Build history of the part. All positions in model axes, mm. Face numbers are marked on the shaded views. A direction names the side the tool comes from. Round coordinates to 2 decimals unless told otherwise and drop trailing zeros. Write each loop counter-clockwise with the first axis right and the second up, starting at its lowest first coordinate (ties: lowest second). Pieces come first, ordered by that corner, then holes. Notation, with made-up numbers: M 16,79 L 43,79 A15 ccw 43,99 Z; hole C -3,-19 d10. An arc over 180 degrees is marked long. Use a Markdown table: item, result.
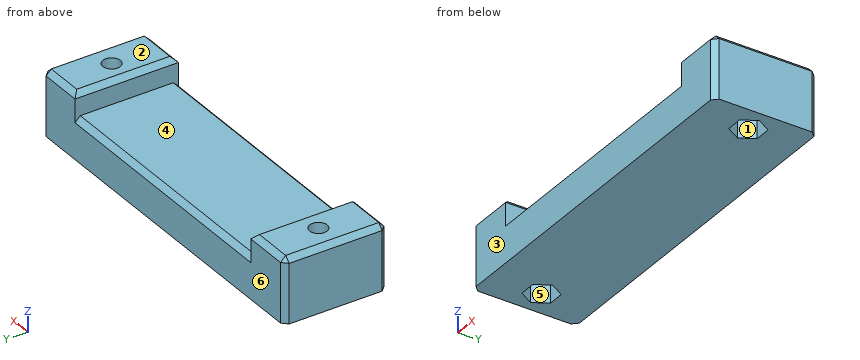
from build123d import *

# Parameters (mm, degrees)
SKETCH023_W     = 70
SKETCH023_H     = 20
PAD012_DEPTH    = 8
SKETCH024_W     = 9.6
SKETCH024_H     = 20
SKETCH024_W_2   = 9.4
PAD013_DEPTH    = 12.5
SKETCH025_R     = 1.7
HOLE003_DEPTH   = 25
POCKET002_DEPTH = 5
CHAMFER004_SIZE = 1


with BuildPart() as part:
    # Sketch023 → Pad012 (new body)
    with BuildSketch(Plane.XY):
        with Locations((0, -110)):
            Rectangle(SKETCH023_W, SKETCH023_H)
    extrude(amount=-PAD012_DEPTH)

    # Sketch024 → Pad013 (join)
    with BuildSketch(Plane.XY.offset(-8)):
        with Locations((-30.2, -110)):
            Rectangle(SKETCH024_W, SKETCH024_H)
        with Locations((30.3, -110)):
            Rectangle(SKETCH024_W_2, SKETCH024_H)
    extrude(amount=PAD013_DEPTH)

    # Sketch025 → Hole003 (cut)
    with BuildSketch(Plane.XY.offset(5)):
        with Locations((-30, -110)):
            Circle(SKETCH025_R)
        with Locations((30, -110)):
            Circle(SKETCH025_R)
    extrude(amount=-HOLE003_DEPTH, mode=Mode.SUBTRACT)

    # Sketch026 → Pocket002 (cut)
    with BuildSketch(Plane.XY.offset(-8)):
        Polygon((-28.412287, -112.75), (-26.824574, -110), (-28.412287, -107.25), (-31.587713, -107.25), (-33.175426, -110), (-31.587713, -112.75), align=None)
        Polygon((31.587713, -112.75), (33.175426, -110), (31.587713, -107.25), (28.412287, -107.25), (26.824574, -110), (28.412287, -112.75), align=None)
    extrude(amount=POCKET002_DEPTH, mode=Mode.SUBTRACT)

    # Chamfer004
    chamfer004_edges = [part.edges().sort_by_distance(p)[0] for p in [
        (-25.4, -110, 4.5),
        (25.6, -110, 4.5),
        (-30.2, -100, 4.5),
        (-35, -110, 4.5),
        (30.3, -100, 4.5),
        (35, -110, 4.5),
        (-30.2, -120, 4.5),
        (30.3, -120, 4.5),
        (0.1, -120, 0),
        (0.1, -100, 0),
        (-35, -120, -4),
        (-35, -100, -4),
        (35, -120, -4),
        (35, -100, -4),
    ]]
    chamfer(chamfer004_edges, length=CHAMFER004_SIZE)


with BuildPart() as part_1:
    # Body003 placement: moved
    add(part.part.moved(Location((0, -25, 0))))


solid = part_1.part
Q1. Cut at A-A on z = 2.75. Give the cut face in (x, y).
Response values:
| item | result |
|---|---|
| outline | M -35,-144 L -34,-145 L -25.4,-145 L -25.4,-125 L -34,-125 L -35,-126 Z; M 25.6,-145 L 34,-145 L 35,-144 L 35,-126 L 34,-125 L 25.6,-125 Z; hole C -30,-135 d3.4; hole C 30,-135 d3.4 |
Q2. Cut at B-B on x = -30. Give the cut face in (y, z), and give its area (3 significant figures).
Response values:
| item | result |
|---|---|
| outline | M -145,-8 L -137.75,-8 L -137.75,-3 L -136.7,-3 L -136.7,4.5 L -144,4.5 L -145,3.5 Z; M -133.3,-3 L -132.25,-3 L -132.25,-8 L -125,-8 L -125,3.5 L -126,4.5 L -133.3,4.5 Z |
| area | 196 mm2 |
Q3. Cut at C-C on z = -7. Give the cut face in (x, y).
Response values:
| item | result |
|---|---|
| outline | M -35,-144 L -34,-145 L 34,-145 L 35,-144 L 35,-126 L 34,-125 L -34,-125 L -35,-126 Z; hole M -33.18,-135 L -31.59,-137.75 L -28.41,-137.75 L -26.82,-135 L -28.41,-132.25 L -31.59,-132.25 Z; hole M 26.82,-135 L 28.41,-137.75 L 31.59,-137.75 L 33.18,-135 L 31.59,-132.25 L 28.41,-132.25 Z |
Q4. Two-plate mould, pull along Y, no slides. Class the marked faces 3, 4, 5 and 6: +Y half, -Y half, draft (parallel to the pull), parting line (faces both ways), or undercut.
Response values:
| item | result |
|---|---|
| face 3 | -Y half |
| face 4 | draft |
| face 5 | undercut |
| face 6 | +Y half |
Q5. Drill centre lines: L1, parallel to X at y = -135, z = 1.75; L2, parallel to X at y = -143, z = 3; L3, parallel to Y at x = 30, z = 1.25. Where is each one in solid material? Low to high.
Response values:
| item | result |
|---|---|
| L1 | x = -35 to -31.7, -28.3 to -25.4, 25.6 to 28.3, 31.7 to 35 |
| L2 | x = -35 to -25.4, 25.6 to 35 |
| L3 | y = -145 to -136.7, -133.3 to -125 |
Q6. Drop flat-ended pins along their axis: P1, Ø5.5, axis at x = -2, y = -131.5, coming from the +Z side; P2, Ø1.6, axis at x = -29.5, y = -134, coming from the -Z side. Give the stop position or say it passes through.
Response values:
| item | result |
|---|---|
| P1 | stops at z = 0 |
| P2 | stops at z = -3 |
Q7. Which spindle directions (+Z, -Z, +X, -X, +Y, -Y) get a long thin tool onto all of the face, cutting with end or side? Do the marked faces 1 and 2. Say none if no direction does.
Response values:
| item | result |
|---|---|
| face 1 | -Z |
| face 2 | +Z, +X, -X, +Y, -Y |
Q8. Cut at D-D on y = -134.25. Give the cut face in (x, z), and give its area (3 significant figures).
Response values:
| item | result |
|---|---|
| outline | M -35,-8 L -32.74,-8 L -32.74,-3 L -31.53,-3 L -31.53,4.5 L -34,4.5 L -35,3.5 Z; M -28.47,-3 L -27.26,-3 L -27.26,-8 L 27.26,-8 L 27.26,-3 L 28.47,-3 L 28.47,4.5 L 26.6,4.5 L 25.6,3.5 L 25.6,0 L -25.4,0 L -25.4,3.5 L -26.4,4.5 L -28.47,4.5 Z; M 31.53,-3 L 32.74,-3 L 32.74,-8 L 35,-8 L 35,3.5 L 34,4.5 L 31.53,4.5 Z |
| area | 543 mm2 |
